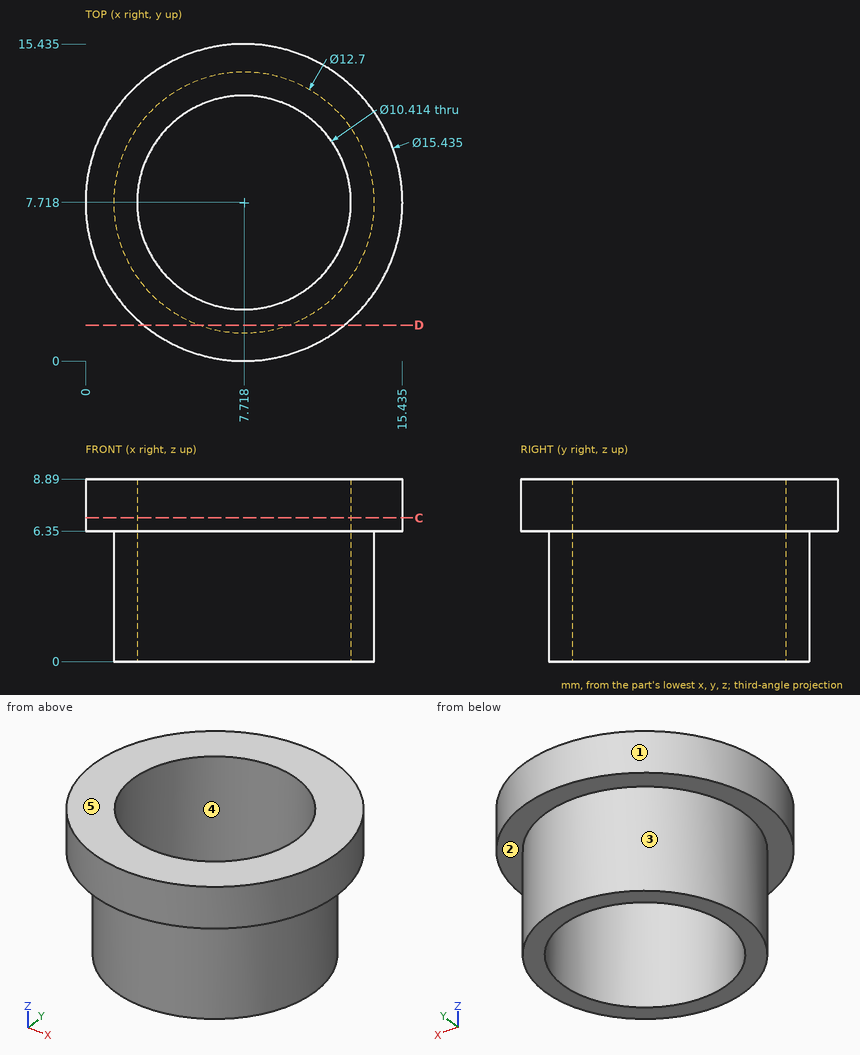
Geometry: see drawing. Coordinates: mm, zero at the bounding-box minimum. A direction names the side the tool comes from. Coordinates: 2 decimals unless noted, no trailing zeros. Loops run counter-clockwise (first coordinate to the right, second up) from the corner with the lowest first, then second, coordinate; pieces in that order, holes last. Notation, with made-up numbers: M 34.25,-33.75 L 58.25,-33.75 A13 cw 58.25,-23.75 Z; hole C 40.5,-29.5 d8. An arc over 180 degrees is marked long. Put each result on its own line as item: value. Start each with the question number.
1) Reachability of the marked faces 1 and 2 from +Z, -Z, +X, -X, +Y, -Y: full face, straight path, thin tool, end or side. Return the list, or none.
2) Ray query, L1, parallel to Y at x = 8.5, z = 4.75 (1 decimal); L2, parallel to X at y = 3, z = 3.5 (1 decimal); L3, parallel to Y at x = 6.75, z = 8 (1 decimal). Return the intervals inside material, ascending. Write a range as from..to.
3) Pull-direction query (Y, two-part tool) for the marked faces 3, 4 and 5; classes: pulls with the +Y half, pulls with the -Y half, needs draft (parallel to the pull), parting line crosses it, or undercut.
4) Cut plane C-C on z = 7. Return the cut outline in (x, y) (1 decimal), then the cut area to 3 significant figures.
5) Cut plane D-D on y = 1.75. Return the cut outline in (x, z).
6) Contact query for flat-ended pins moving along their axis: pin 1 Ø4 at (y, z) = (2, 3) entering from -X; pin 2 Ø5 at (x, z) = (1.5, 2) entering from -Y; pin 3 Ø3 at (x, z) = (6, 4.5) entering from -Y. Output: stop coordinate, or through.
The answers:
1. face 1: +Z, -Z
1. face 2: -Z
2. L1: y = 1.4..2.6, 12.9..14
2. L2: x = 3.5..5.5, 9.9..12
2. L3: y = 0.1..2.6, 12.8..15.4
3. face 3: parting line crosses it
3. face 4: undercut
3. face 5: needs draft
4. outline: C 7.7,7.7 d15.4; hole C 7.7,7.7 d10.4
4. area: 102 mm²
5. outline: M 2.82,6.35 L 5.55,6.35 L 5.55,0 L 9.89,0 L 9.89,6.35 L 12.61,6.35 L 12.61,8.89 L 2.82,8.89 Z
6. pin 1: stops at x = 2.57
6. pin 2: stops at y = 2.57
6. pin 3: stops at y = 1.37
